from build123d import *

# Parameters (mm, degrees)
CYLINDER007_R     = 1.5
CYLINDER007_DEPTH = 30
CYLINDER006_R     = 1.5
CYLINDER006_DEPTH = 30
CYLINDER005_R     = 1.5
CYLINDER005_DEPTH = 30
CYLINDER004_R     = 1.5
CYLINDER004_DEPTH = 30
CYLINDER003_R     = 1.5
CYLINDER003_DEPTH = 30
CYLINDER002_R     = 1.5
CYLINDER002_DEPTH = 30
CYLINDER001_R     = 1.5
CYLINDER001_DEPTH = 30
CYLINDER_R        = 1.5
CYLINDER_DEPTH    = 30
BOX003_W          = 10
BOX003_H          = 10
BOX003_DEPTH      = 10
BOX004_W          = 80
BOX004_H          = 10
BOX004_DEPTH      = 10
BOX002_W          = 10
BOX002_H          = 10
BOX002_DEPTH      = 10
BOX001_W          = 190
BOX001_H          = 190
BOX001_DEPTH      = 45
BOX_W             = 200
BOX_H             = 200
BOX_DEPTH         = 50


with BuildPart() as cylinder007:
    # Cylinder007 → Cylinder007 (new body)
    with BuildSketch(Plane(origin=(34.06, 110.24, 0), x_dir=(1, 0, 0), z_dir=(0, 0, 1))):
        Circle(CYLINDER007_R)
    extrude(amount=CYLINDER007_DEPTH)


with BuildPart() as cylinder006:
    # Cylinder006 → Cylinder006 (new body)
    with BuildSketch(Plane(origin=(34.06, 174.24, 0), x_dir=(1, 0, 0), z_dir=(0, 0, 1))):
        Circle(CYLINDER006_R)
    extrude(amount=CYLINDER006_DEPTH)


with BuildPart() as cylinder005:
    # Cylinder005 → Cylinder005 (new body)
    with BuildSketch(Plane(origin=(72.56, 174.24, 0), x_dir=(1, 0, 0), z_dir=(0, 0, 1))):
        Circle(CYLINDER005_R)
    extrude(amount=CYLINDER005_DEPTH)


with BuildPart() as cylinder004:
    # Cylinder004 → Cylinder004 (new body)
    with BuildSketch(Plane(origin=(72.56, 110.24, 0), x_dir=(1, 0, 0), z_dir=(0, 0, 1))):
        Circle(CYLINDER004_R)
    extrude(amount=CYLINDER004_DEPTH)


with BuildPart() as cylinder003:
    # Cylinder003 → Cylinder003 (new body)
    with BuildSketch(Plane(origin=(178.89, 102.19, 0), x_dir=(1, 0, 0), z_dir=(0, 0, 1))):
        Circle(CYLINDER003_R)
    extrude(amount=CYLINDER003_DEPTH)


with BuildPart() as cylinder002:
    # Cylinder002 → Cylinder002 (new body)
    with BuildSketch(Plane(origin=(178.89, 178.19, 0), x_dir=(1, 0, 0), z_dir=(0, 0, 1))):
        Circle(CYLINDER002_R)
    extrude(amount=CYLINDER002_DEPTH)


with BuildPart() as cylinder001:
    # Cylinder001 → Cylinder001 (new body)
    with BuildSketch(Plane(origin=(111.89, 178.19, 0), x_dir=(1, 0, 0), z_dir=(0, 0, 1))):
        Circle(CYLINDER001_R)
    extrude(amount=CYLINDER001_DEPTH)


with BuildPart() as cylinder:
    # Cylinder → Cylinder (new body)
    with BuildSketch(Plane(origin=(111.89, 102.19, 0), x_dir=(1, 0, 0), z_dir=(0, 0, 1))):
        Circle(CYLINDER_R)
    extrude(amount=CYLINDER_DEPTH)


with BuildPart() as cube003:
    # Box003 → Box003 (new body)
    with BuildSketch(Plane(origin=(191, 106.5, 15), x_dir=(1, 0, 0), z_dir=(0, 0, 1))):
        with Locations((5, 5)):
            Rectangle(BOX003_W, BOX003_H)
    extrude(amount=BOX003_DEPTH)


with BuildPart() as cube004:
    # Box004 → Box004 (new body)
    with BuildSketch(Plane(origin=(100, -1, 25), x_dir=(1, 0, 0), z_dir=(0, 0, 1))):
        with Locations((40, 5)):
            Rectangle(BOX004_W, BOX004_H)
    extrude(amount=BOX004_DEPTH)


with BuildPart() as fusion:
    # Box002 → Box002 (new body)
    with BuildSketch(Plane(origin=(138, 190.5, 20), x_dir=(1, 0, 0), z_dir=(0, 0, 1))):
        with Locations((5, 5)):
            Rectangle(BOX002_W, BOX002_H)
    extrude(amount=BOX002_DEPTH)

    # Fusion: union Cube003, Cube004
    add(cube003.part)
    add(cube004.part)


with BuildPart() as cube001:
    # Box001 → Box001 (new body)
    with BuildSketch(Plane(origin=(5, 5, 5), x_dir=(1, 0, 0), z_dir=(0, 0, 1))):
        with Locations((95, 95)):
            Rectangle(BOX001_W, BOX001_H)
    extrude(amount=BOX001_DEPTH)


with BuildPart() as box_bottom:
    # Box → Box (new body)
    with BuildSketch(Plane.XY):
        with Locations((100, 100)):
            Rectangle(BOX_W, BOX_H)
    extrude(amount=BOX_DEPTH)

    # Cut: cut Cube001
    add(cube001.part, mode=Mode.SUBTRACT)

    # Cut001: cut Fusion
    add(fusion.part, mode=Mode.SUBTRACT)

    # Fusion001: union Cylinder007, Cylinder006, Cylinder005, Cylinder004, Cylinder003, Cylinder002, Cylinder001, Cylinder
    add(cylinder007.part)
    add(cylinder006.part)
    add(cylinder005.part)
    add(cylinder004.part)
    add(cylinder003.part)
    add(cylinder002.part)
    add(cylinder001.part)
    add(cylinder.part)


solid = box_bottom.part
Model file for the job. Use its own axes, mm. A direction names the side the tool comes from. Give positions to 0.01 mm unless a question says otherwise; leave off trailing zeros. Order: outer loops, then holes, each group sorted by start corner. A loop starts at its lowest first (then second) coordinate and runs counter-clockwise, first axis right, second up. Notation, with made-up numbers: M 88.25,74.25 L 123.25,74.25 A14 cw 123.25,91.25 Z; hole C 1.5,34 d11. An arc over 180 degrees is marked long. Put each result on its own line as item: value. Start each with the question number.
(1) Band-saw the part on A-A on z = 17.5. Count the separate pieces of the cut face and the enclosed holes in it, then the cut area to 3 significant figures.
(2) Pin check, flat tip, straight feed: pin 1 Ø1.5 at (x, y) = (179, 178) entering from +Z. Stop position of the tip, or through.
(3) Band-saw the part on D-D on z = 39. Give the cut face in (x, y).
(4) Drill centre lines: L1, parallel to X at y = 46, z = 43; L2, parallel to Z at x = 159, y = 169. Where is each one in solid material? Low to high. Write a range as [from, to].
(5) Tool access for faces 4 (the face through (143, 198, 30)), 5 (the face through (100, 2, 30)), 6 (the face through (143, 198, 20)), 7 (the face through (99, 195, 27)): list every direction of +Z, -Z, +X, -X, +Y, -Y with a clear straight run to the whole face (end or side of a thin tool).
(6) Band-saw the part on C-C on y = 61. Give the cut face in (x, z).
(7) Band-saw the part on B-B on x = 117. Give the cut face in (y, z).
(8) Pull direction X, two halves, no side cores. Call faces 1 (the face through (138, 197, 25)), 2 (the face through (99, 101, 0)), 3 (the face through (200, 99, 25)): released by +X, released by -X, zero draft, split by the parting line, or undercut.
Results below:
1. separate pieces: 9
1. enclosed holes: 0
1. area: 3,910 mm2
2. pin 1: stops at z = 30
3. outline: M 0,0 L 200,0 L 200,200 L 0,200 Z; hole M 5,5 L 195,5 L 195,195 L 5,195 Z
4. L1: x = [0, 5], [195, 200]
4. L2: z = [0, 5]
5. face 4: +Y, -Y
5. face 5: -Y
5. face 6: +Y
5. face 7: +Z
6. outline: M 0,0 L 200,0 L 200,50 L 195,50 L 195,5 L 5,5 L 5,50 L 0,50 Z
7. outline: M 0,0 L 200,0 L 200,50 L 195,50 L 195,5 L 5,5 L 5,25 L 0,25 Z; M 0,35 L 5,35 L 5,50 L 0,50 Z
8. face 1: undercut
8. face 2: zero draft
8. face 3: released by +X
